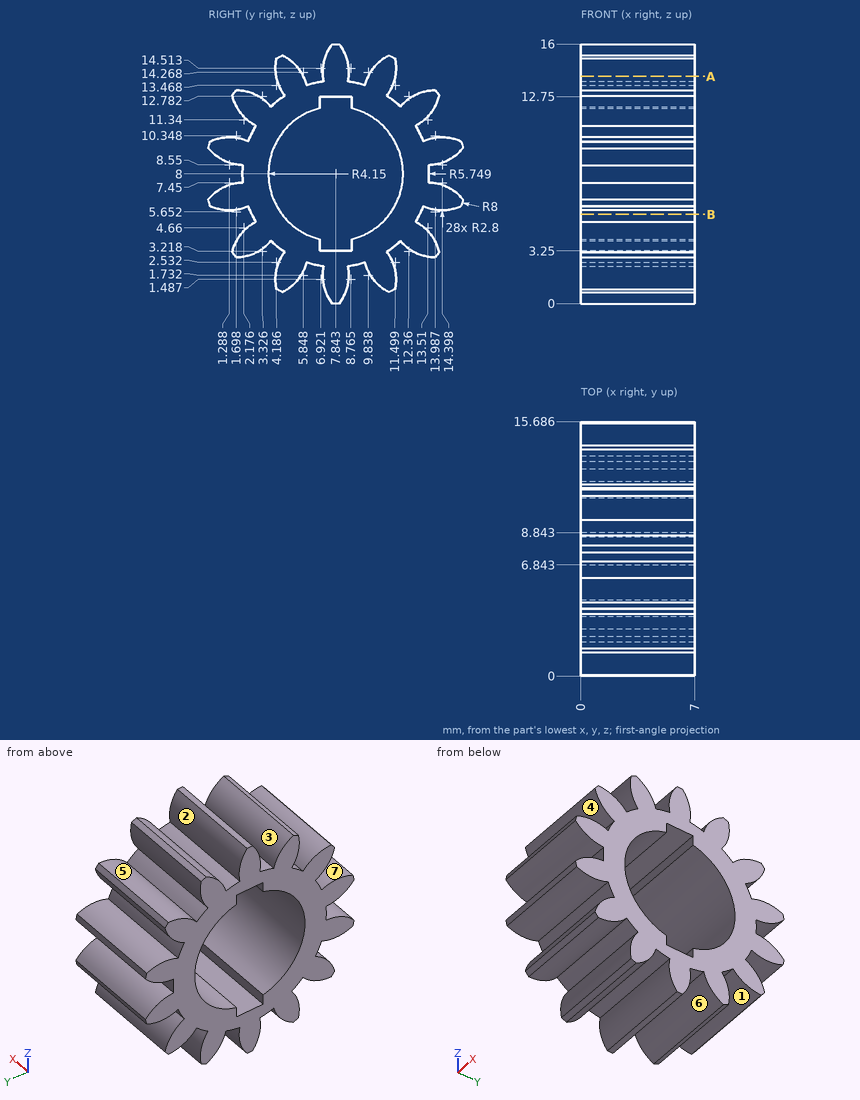
Drawing for the job (mm, zero at the part's lowest x, y, z). A direction names the side the tool comes from. Coordinates: 2 decimals unless noted, no trailing zeros. Order: outer loops, then holes, each group sorted by start corner. A loop starts at its lowest first (then second) coordinate and runs counter-clockwise, first axis right, second up. Notation, with made-up numbers: (46, 49.5) - (58, 49.5) arc R19 ccw to (58, 80.5) - close; hole circle Ø9 at (-39.75, -26.75). An arc over 180 degrees is marked (long way). Use a Markdown table: item, result. Add a question column.
(1) Drill centre lines: line 1 along Z through (x, y) = (1.25, 8); line 2 along Z through (x, y) = (1.5, 13) (1 decimal); line 3 along Y through (x, z) = (1.75, 11) (1 decimal). Where is each one in solid material? Low to high. Write a range as [from, to].
(2) Flat gauge pins, fed straight in: pin 1 (0.8 mm diameter, centred on x = 3.5, z = 3.5, fed in from -Y); pin 2 (2 mm diameter, centred on x = 3, z = 14, fed in from +Y); pin 3 (0.8 mm diameter, centred on x = 2, z = 12.5, fed in from +Y) (1 decimal); pin 4 (3 mm diameter, centred on x = 6.5, y = 9.5, fed in from +Z). Where does each tip first touch, or does it go through?
(3) Which spindle directions (+Z, -Z, +X, -X, +Y, -Y) get a long thin tool onto all of the face, cutting with end or side? Do the marked faces 1, 2, 3 and 4. Say none if no direction does.
(4) Pull direction Z, two halves, no side cores. Call the marked faces 5, 6 and 7: +Z half, -Z half, draft (parallel to the pull), parting line (faces both ways), or undercut.
(5) Saw through at B-B (z = 5.5). Give the cut face in (x, y) (1 decimal).
(6) Saw through at A-A (z = 14). Count the separate pieces of the cut face and the enclosed holes in it.
Solved:
| question | item | result |
|---|---|---|
| 1 | line 1 | z = [0, 3.25], [12.75, 16] |
| 1 | line 2 | z = [3, 4.9], [5.5, 10.5], [11.1, 13] |
| 1 | line 3 | y = [2.9, 5], [10.7, 12.8] |
| 2 | pin 1 | stops at y = 1.46 |
| 2 | pin 2 | stops at y = 14.09 |
| 2 | pin 3 | stops at y = 14.2 |
| 2 | pin 4 | stops at z = 16 |
| 3 | face 1 | -Z, +X, -X |
| 3 | face 2 | +X, -X |
| 3 | face 3 | +Z, +X, -X |
| 3 | face 4 | +X, -X, -Y |
| 4 | face 5 | +Z half |
| 4 | face 6 | -Z half |
| 4 | face 7 | undercut |
| 5 | outline | (0, 2.7) - (7, 2.7) - (7, 4.5) - (0, 4.5) - close; (0, 11.2) - (7, 11.2) - (7, 13) - (0, 13) - close |
| 6 | separate pieces | 3 |
| 6 | enclosed holes | 0 |
